Could you check a few things on this model? Use its own coordinates, in mm. A direction names the side the tool comes from. Coordinates: 2 decimals unless noted, no trailing zeros. Loops run counter-clockwise (first coordinate to the right, second up) from the corner with the lowest first, then second, coordinate; pieces in that order, holes last.
1) Imagine slicing it at D-D on z = 85.5. Please give me the cut outline in (x, y), plus the area to 3 significant figures.
2) Imagine slicing it at A-A on x = 81.5. Please give me the cut outline in (y, z).
3) For faces 1 (the face through (50, 45, 70)), 2 (the face through (3.884, 8.062, 24.65)), which set-ups out of +Z, -Z, +X, -X, +Y, -Y let a thin tool reach every point of the face, with its end or its side?
4) Imagine slicing it at C-C on y = 48.5. Please give me the cut outline in (x, z).
5) Thinking about a two-plate mould opening in X: for faces 3 (the face through (97.466, 82.191, 24.65)), 4 (the face through (0, 46, 25)), 5 (the face through (24.31, 21.31, 74.65)), which applies, released by +X, released by -X, zero draft, split by the parting line, or undercut?
6) Will these pins go through, and if not, where does the flat tip stop? P1, Ø13, axis at x = 95.88, y = 4.21, coming from the +Z side; P2, Ø3, axis at x = 65, z = 74, coming from the +Y side; P3, Ø4, axis at y = 69, z = 52.5, coming from the +X side.
7) If I drill on line 1 along Z through (x, y) = (77, 83.5); line 2 along X through (y, z) = (84, 49.5); line 3 along Y through (x, z) = (25.5, 81.5), over which ranges is the centre line in solid material (lowest first)?
8) Imagine slicing it at B-B on z = 22. Please give me the cut outline in (x, y).
Autodesk Inventor part; units mm, degrees
ref_plane "YZ Plane" through (0, 0, 0) normal (1, 0, 0) x (0, 1, 0)
ref_plane "XZ Plane" through (0, 0, 0) normal (0, 1, 0) x (-1, 0, 0)
ref_plane "XY Plane" through (0, 0, 0) normal (0, 0, 1) x (1, 0, 0)
sketch "Boceto1" plane through (0, 0, 0) normal (0, 0, 1) x (1, 0, 0)
  line L0 (2, 0) -> (98, 0)
  line L1 (100, 2) -> (100, 88)
  line L2 (98.0371, 89.9629) -> (1.9629, 89.9629)
  line L3 (0, 88) -> (0, 2)
  arc A0 (1.9629, 89.9629) -> (0, 88) centre (1.9629, 88) ccw
  arc A1 (100, 88) -> (98.0371, 89.9629) centre (98.0371, 88) ccw
  arc A2 (0, 2) -> (2, 0) centre (2, 2) ccw
  arc A3 (98, 0) -> (100, 2) centre (98, 2) ccw
  circle A4 centre (4, 85.9629) radius 4
  circle A5 centre (96, 85.9629) radius 4
  circle A6 centre (4, 4) radius 4
  circle A7 centre (96, 4) radius 4
  point P0 (0, 0)
  point P1 (100, 89.9629)
  point P2 (100, 0)
  point P3 (0, 89.9629)
  dimension "d0" = 100
  dimension "d6" = 8
  dimension "d7" = 8
  dimension "d8" = 8
  dimension "d9" = 8
extrude "Extrusión1" add sketch "Boceto1" along normal blind 50
sketch "Boceto2" plane through (0, 0, 50) normal (0, 0, 1) x (1, 0, 0)
  circle A0 centre (4.1038, 85.8268) radius 4
  circle A1 centre (95.7307, 85.8268) radius 4
  point P0 (0, 0)
  dimension "d12" = 8
  dimension "d13" = 8
hole "Agujero1" at (4.1038, 85.8268, 50) direction (0, 0, -1) diameter 8 end through all
sketch "Boceto3" plane through (0, 0, 50) normal (0, 0, 1) x (1, 0, 0)
  circle A0 centre (95.9335, 85.8863) radius 4
  point P0 (0, 0)
  dimension "d21" = 8
hole "Agujero2" at (95.9335, 85.8863, 50) direction (0, 0, -1) diameter 8 end through all
sketch "Boceto4" plane through (0, 0, 50) normal (0, 0, 1) x (1, 0, 0)
  circle A0 centre (95.8814, 4.2134) radius 4
  point P0 (0, 0)
  dimension "d29" = 8
hole "Agujero3" at (95.8814, 4.2134, 50) direction (0, 0, -1) diameter 8 end through all
sketch "Boceto5" plane through (0, 0, 50) normal (0, 0, 1) x (1, 0, 0)
  circle A0 centre (4.0599, 4.0663) radius 4
  point P0 (0, 0)
  dimension "d37" = 8
hole "Agujero4" at (4.0599, 4.0663, 50) direction (0, 0, -1) diameter 8 end through all
sketch "Boceto6" plane through (0, 0, 50) normal (0, 0, 1) x (1, 0, 0)
  circle A0 centre (50.1065, 44.9629) radius 35
  line L0 (98.0371, 89.9629) -> (1.9629, 89.9629)
  line L1 (2, 0) -> (98, 0)
  circle A1 centre (50.1065, 44.9629) radius 30
  point P0 (0, 0)
  point P1 (50, 89.9629)
  point P2 (50, 0)
  dimension "d45" = 70
  dimension "d48" = 60
extrude "Extrusión2" add sketch "Boceto6" along normal blind 50
sketch "Boceto7" plane through (50.1065, 44.9629, 50) normal (0, 0, 1) x (1, 0, 0)
  circle A0 centre (0, 0) radius 30
  point P0 (-50.1065, -44.9629)
  dimension "d51" = 60
extrude "Extrusión3" add sketch "Boceto7" along normal blind 20
properties part number "dinamica T1"
Filled in:
1. outline: circle Ø70 at (50.11, 44.96); hole circle Ø60 at (50.11, 44.96)
1. area: 1,020 mm2
2. outline: (0, 0) - (89.96, 0) - (89.96, 50) - (60.44, 50) - (60.44, 100) - (29.49, 100) - (29.49, 50) - (0, 50) - close
3. face 1: +Z
3. face 2: +Z, -Z
4. outline: (0, 0) - (100, 0) - (100, 50) - (84.93, 50) - (84.93, 100) - (79.9, 100) - (79.9, 70) - (20.32, 70) - (20.32, 100) - (15.29, 100) - (15.29, 50) - (0, 50) - close
5. face 3: undercut
5. face 4: released by -X
5. face 5: split by the parting line
6. P1: stops at z = 50
6. P2: stops at y = 77.3
6. P3: stops at x = 77.3
7. line 1: z = 0 to 50
7. line 2: x = 0 to 0.55, 7.66 to 92.41, 99.46 to 100
7. line 3: y = 20.07 to 27.8, 62.12 to 69.85
8. outline: (0, 2) arc R2 ccw to (2, 0) - (98, 0) arc R2 ccw to (100, 2) - (100, 88) arc R1.96 ccw to (98.04, 89.96) - (1.96, 89.96) arc R1.96 ccw to (0, 88) - close; hole circle Ø8 at (4.06, 4.07); hole circle Ø8 at (4.1, 85.83); hole circle Ø8 at (95.88, 4.21); hole circle Ø8 at (95.93, 85.89)
